The model under review builds one solid part; all positions refer to its coordinate system, in mm. Face numbers are marked on the shaded views. A direction names the side the tool comes from. Coordinates: 2 decimals unless noted, no trailing zeros. Order: outer loops, then holes, each group sorted by start corner. A loop starts at its lowest first (then second) coordinate and runs counter-clockwise, first axis right, second up.
```python
from build123d import *

# Parameters (mm, degrees)
ESQUISSE1_R        = 1.35
ESQUISSE1_R_2      = 1.5
BOSS_EXTRU_1_DEPTH = 4.9


with BuildPart() as part:
    # Esquisse1 → Boss.-Extru.1 (new body)
    with BuildSketch(Plane.XY.offset(377.0447)):
        Polygon((15.891185209, 3.330523996), (17.295074786, 4.667009593), (18.397064454, 6.110993158), (19.198464212, 7.515709734), (19.829414022, 9.236036216), (20.160733922, 11.107826651), (20.275133888, 13.944835796), (20.111733937, 17.038324864), (19.548124107, 22.181683313), (19.336824171, 24.193402707), (19.277384189, 26.157782114), (19.497574122, 27.722941643), (20.015153966, 29.300491167), (20.842573717, 30.928140676), (21.916433393, 32.504840201), (23.323482969, 34.1655297), (23.323482969, 35.665529248), (26.499992011, 35.665529248), (27.249991785, 35.866489188), (27.79903162, 36.415529022), (27.999991559, 37.165528796), (27.999991559, 47.499985681), (27.933001579, 47.749985605), (27.749991634, 47.93299555), (27.49999171, 47.99998553), (1.999999397, 47.99998553), (1.234632628, 47.847745576), (0.585786323, 47.414205706), (0.152240954, 46.765355902), (0, 45.999986133), (0, 44.499986585), (0.06698734, 44.24998666), (0.249999925, 44.066976716), (0.499999949, 43.999986736), (7.749997664, 43.999986736), (7.783491654, 44.124986698), (7.874997626, 44.21649667), (7.999997588, 44.24998666), (8.124997551, 44.21649667), (8.216504523, 44.124986698), (8.249997513, 43.999986736), (8.216504523, 43.874986773), (8.124997551, 43.783476801), (7.999997588, 43.749986811), (7.999997588, 39.249988168), (8.124997551, 39.216498178), (8.216504523, 39.124988205), (8.249997513, 38.999988243), (8.216504523, 38.874988281), (8.124997551, 38.783478308), (7.999997588, 38.749988318), (7.874997626, 38.783478308), (7.783491654, 38.874988281), (7.749997664, 38.999988243), (0.499999949, 38.999988243), (0.249999925, 38.932998263), (0.06698734, 38.749988318), (0, 38.499988394), (0, 33.99998975), (0.06698734, 33.749989826), (0.249999925, 33.566979881), (0.499999949, 33.499989901), (7.749997664, 33.499989901), (7.783491654, 33.624989863), (7.874997626, 33.716499836), (7.999997588, 33.749989826), (8.124997551, 33.716499836), (8.216504523, 33.624989863), (8.249997513, 33.499989901), (8.216504523, 33.374989939), (8.124997551, 33.283479966), (7.999997588, 33.249989976), (7.999997588, 28.749991333), (8.124997551, 28.716501343), (8.216504523, 28.624991371), (8.249997513, 28.499991408), (8.216504523, 28.374991446), (8.124997551, 28.283481474), (7.999997588, 28.249991484), (7.874997626, 28.283481474), (7.783491654, 28.374991446), (7.749997664, 28.499991408), (0.499999949, 28.499991408), (0.249999925, 28.433001429), (0.06698734, 28.249991484), (0, 27.999991559), (0, 23.499992916), (0.06698734, 23.249992991), (0.249999925, 23.066983046), (0.499999949, 22.999993066), (7.749997664, 22.999993066), (7.783491654, 23.124993029), (7.874997626, 23.216503001), (7.999997588, 23.249992991), (8.124997551, 23.216503001), (8.216504523, 23.124993029), (8.249997513, 22.999993066), (8.216504523, 22.874993104), (8.124997551, 22.783483132), (7.999997588, 22.749993142), (7.999997588, 18.249994498), (8.124997551, 18.216504508), (8.216504523, 18.124994536), (8.249997513, 17.999994574), (8.216504523, 17.874994611), (8.124997551, 17.783484639), (7.999997588, 17.749994649), (7.874997626, 17.783484639), (7.783491654, 17.874994611), (7.749997664, 17.999994574), (0.499999949, 17.999994574), (0.249999925, 17.933004594), (0.06698734, 17.749994649), (0, 17.499994724), (0, 12.999996081), (0.06698734, 12.749996156), (0.249999925, 12.566986212), (0.499999949, 12.499996232), (7.749997664, 12.499996232), (7.783491654, 12.624996194), (7.874997626, 12.716506166), (7.999997588, 12.749996156), (8.124997551, 12.716506166), (8.216504523, 12.624996194), (8.249997513, 12.499996232), (8.216504523, 12.374996269), (8.124997551, 12.283486297), (7.999997588, 12.249996307), (7.999997588, 7.749997664), (8.124997551, 7.716503674), (8.216504523, 7.624997701), (8.249997513, 7.499997739), (8.216504523, 7.374997777), (8.124997551, 7.283491804), (7.999997588, 7.249997814), (7.874997626, 7.283491804), (7.783491654, 7.374997777), (7.749997664, 7.499997739), (0.499999949, 7.499997739), (0.249999925, 7.433009759), (0.06698734, 7.249997814), (0, 6.99999789), (0, 1.999999397), (0.152240954, 1.234632628), (0.585786323, 0.585786223), (1.234632628, 0.152240854), (1.999999397, 0), (3.776477862, 0.025545672), (7.248430815, 0.262472121), (10.036716974, 0.718076284), (12.321666285, 1.373609586), (14.238535708, 2.233213327), align=None)
        with Locations((21.999992961, 41.999982339)):
            Circle(ESQUISSE1_R, mode=Mode.SUBTRACT)
        with Locations((9.99999793, 25.749992786)):
            Circle(ESQUISSE1_R_2, mode=Mode.SUBTRACT)
        Polygon((12.933006101, 13.249996006), (12.749996156, 13.066986061), (12.499996232, 12.999996081), (11.499996533, 12.999996081), (11.249996609, 13.066986061), (11.066986664, 13.249996006), (10.999996684, 13.49999593), (10.999996684, 16.999994875), (11.066986664, 17.2499948), (11.249996609, 17.433004745), (11.499996533, 17.499994724), (12.499996232, 17.499994724), (12.749996156, 17.433004745), (12.933006101, 17.2499948), (12.999996081, 16.999994875), (12.999996081, 13.49999593), align=None, mode=Mode.SUBTRACT)
        Polygon((11.249996609, 34.06697973), (11.066986664, 34.249989675), (10.999996684, 34.4999896), (10.999996684, 37.999988544), (11.066986664, 38.249988469), (11.249996609, 38.432998414), (11.499996533, 38.499988394), (12.499996232, 38.499988394), (12.749996156, 38.432998414), (12.933006101, 38.249988469), (12.999996081, 37.999988544), (12.999996081, 34.4999896), (12.933006101, 34.249989675), (12.749996156, 34.06697973), (12.499996232, 33.99998975), (11.499996533, 33.99998975), align=None, mode=Mode.SUBTRACT)
    extrude(amount=-BOSS_EXTRU_1_DEPTH)


solid = part.part
```
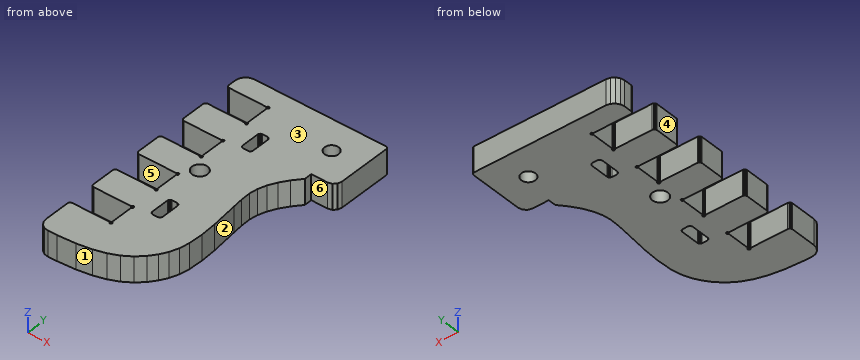
(1) We need section A-A, the plane x = 2.75. Write out the cut boundary in (y, z).
A:
outline: (0.01, 372.14) - (7.5, 372.14) - (7.5, 377.04) - (0.01, 377.04) - close; (12.5, 372.14) - (18, 372.14) - (18, 377.04) - (12.5, 377.04) - close; (23, 372.14) - (28.5, 372.14) - (28.5, 377.04) - (23, 377.04) - close; (33.5, 372.14) - (39, 372.14) - (39, 377.04) - (33.5, 377.04) - close; (44, 372.14) - (48, 372.14) - (48, 377.04) - (44, 377.04) - close
(2) Draft analysis for pull direction Y (two halves, no side actions). For the marked faces 1, 2 and 3, state which applies: released by +Y, released by -Y, zero draft, split by the parting line, or undercut.
A:
face 1: released by -Y
face 2: undercut
face 3: zero draft
(3) We need section B-B, the plane z = 374.75. Count the separate pieces of the cut face and the enclosed holes in it, and give its area (3 significant figures).
A:
separate pieces: 1
enclosed holes: 4
area: 837 mm2
(4) Machinability: for the marked faces 4, 5 and 6, which of the approach directions +Z, -Z, +X, -X, +Y, -Y give a long, thin tool a straight path to every point of the face, cutting with its end or side? Answer none if there is none.
A:
face 4: +Z, -Z, -X, +Y, -Y
face 5: +Z, -Z, -X
face 6: +Z, -Z, +X, -Y
(5) For pin 1 Ø1 at (y, z) = (22, 376) entering from +X; pin 2 Ø0.8 at (x, z) = (12, 374.5) entering from -Y; pin 3 Ø12 at (x, y) = (10.5, 25.5) entering from +Z; pin 4 Ø2 at (y, z) = (31, 376.5) entering from +X, all flat-tipped, find the tip position at first contact; note any pin that passes through.
A:
pin 1: stops at x = 19.62
pin 2: stops at y = 1.17
pin 3: stops at z = 377.04
pin 4: stops at x = 21.57
(6) We need section C-C, the plane y = 20. Write out the cut boundary in (x, z).
A:
outline: (8, 372.14) - (19.79, 372.14) - (19.79, 377.04) - (8, 377.04) - close
(7) Wall thickness on probe 1 along Y at (x, z) = (7.25, 373.8); probe 2 along X at (y, z) = (35, 376.3); probe 3 along Y at (x, z) = (1.5, 375.55): over which ranges is each line inside the solid? List them lowest first.
A:
probe 1: y = 0.26 to 7.5, 12.5 to 18, 23 to 28.5, 33.5 to 39, 44 to 48
probe 2: x = 0 to 11, 13 to 23.32
probe 3: y = 0.1 to 7.5, 12.5 to 18, 23 to 28.5, 33.5 to 39, 44 to 47.9
